The listing builds one solid part. Answer for the finished solid, in the listing's coordinates (mm). A direction names the side the tool comes from. Coordinates: 2 decimals unless noted, no trailing zeros. Order: outer loops, then holes, each group sorted by start corner. A loop starts at its lowest first (then second) coordinate and runs counter-clockwise, first axis right, second up.
from build123d import *

# Parameters (mm, degrees)
SKETCH_W        = 116
SKETCH_H        = 42
PAD_DEPTH       = 42
SKETCH005_W     = 110
SKETCH005_H     = 36
POCKET_DEPTH    = 35
SKETCH006_R     = 1.75
SKETCH006_R_2   = 15
POCKET001_DEPTH = 7.001
POCKET002_DEPTH = 5
SKETCH007_R     = 13
POCKET003_DEPTH = 42.001
SKETCH008_R     = 14
POCKET004_DEPTH = 116.001
SKETCH012_R     = 4
POCKET005_DEPTH = 5
SKETCH013_R     = 4
POCKET006_DEPTH = 5


with BuildPart() as part:
    # Sketch → Pad (new body)
    with BuildSketch(Plane.XZ):
        with Locations((0, 21)):
            Rectangle(SKETCH_W, SKETCH_H)
    extrude(amount=PAD_DEPTH)

    # Sketch005 → Pocket (cut)
    with BuildSketch(Plane(origin=(0, 0, 42), x_dir=(-1, 0, 0), z_dir=(0, 0, 1))):
        with Locations((0, 21)):
            Rectangle(SKETCH005_W, SKETCH005_H)
    extrude(amount=-POCKET_DEPTH, mode=Mode.SUBTRACT)

    # Sketch006 → Pocket001 (cut, through all)
    with BuildSketch(Plane(origin=(0, 0, 7), x_dir=(-1, 0, 0), z_dir=(0, 0, 1))):
        with Locations((-40, 33.5)):
            Circle(SKETCH006_R)
        with Locations((40, 33.5)):
            Circle(SKETCH006_R)
        with Locations((-40, 9)):
            Circle(SKETCH006_R)
        with Locations((40, 9)):
            Circle(SKETCH006_R)
        with Locations((-20, 21)):
            Circle(SKETCH006_R_2)
        with Locations((20, 21)):
            Circle(SKETCH006_R_2)
    extrude(amount=-POCKET001_DEPTH, mode=Mode.SUBTRACT)

    # Sketch011 → Pocket002 (cut)
    with BuildSketch(Plane(origin=(0, 0, 7), x_dir=(-1, 0, 0), z_dir=(0, 0, 1))):
        Polygon((-42.373287, 37.679591), (-37.615921, 37.679591), (-35.237238, 33.559591), (-37.615921, 29.439591), (-42.373287, 29.439591), (-44.75197, 33.559591), align=None)
        Polygon((37.627177, 37.64135), (42.384544, 37.64135), (44.763227, 33.52135), (42.384544, 29.40135), (37.627177, 29.40135), (35.248494, 33.52135), align=None)
        Polygon((37.575129, 13.14135), (42.332495, 13.14135), (44.711178, 9.02135), (42.332495, 4.90135), (37.575129, 4.90135), (35.196446, 9.02135), align=None)
        Polygon((-42.367844, 13.179591), (-37.610478, 13.179591), (-35.231795, 9.059591), (-37.610478, 4.939591), (-42.367844, 4.939591), (-44.746527, 9.059591), align=None)
    extrude(amount=-POCKET002_DEPTH, mode=Mode.SUBTRACT)

    # Sketch007 → Pocket003 (cut, through all)
    with BuildSketch(Plane(origin=(0, 0, 0), x_dir=(1, 0, 0), z_dir=(0, 1, 0))):
        with Locations((-24, -25)):
            Circle(SKETCH007_R)
        with Locations((7, -25)):
            Circle(SKETCH007_R)
        with Locations((38, -25)):
            Circle(SKETCH007_R)
        with BuildLine():
            ThreePointArc((-43, -16.999991), (-48, -12), (-53, -16.999992))
            Line((-53, -16.999992), (-53, -33.999979))
            ThreePointArc((-53, -33.999979), (-48, -39), (-43, -33.999978))
            Line((-43, -16.999991), (-43, -33.999978))
        make_face()
    extrude(amount=-POCKET003_DEPTH, mode=Mode.SUBTRACT)

    # Sketch008 → Pocket004 (cut, through all)
    with BuildSketch(Plane(origin=(-58, 0, 0), x_dir=(0, 0, -1), z_dir=(-1, 0, 0))):
        with Locations((-23, 22)):
            Circle(SKETCH008_R)
    extrude(amount=-POCKET004_DEPTH, mode=Mode.SUBTRACT)

    # Sketch012 → Pocket005 (cut)
    with BuildSketch(Plane(origin=(0, 0, 0), x_dir=(1, 0, 0), z_dir=(0, 1, 0))):
        with Locations((-10, 0)):
            Circle(SKETCH012_R)
        with Locations((10, 0)):
            Circle(SKETCH012_R)
    extrude(amount=-POCKET005_DEPTH, mode=Mode.SUBTRACT)

    # Sketch013 → Pocket006 (cut)
    with BuildSketch(Plane.XZ.offset(42)):
        with Locations((-10, 0)):
            Circle(SKETCH013_R)
        with Locations((10, 0)):
            Circle(SKETCH013_R)
    extrude(amount=-POCKET006_DEPTH, mode=Mode.SUBTRACT)


solid = part.part
1) Section C-C (z = 32.5) is taken. Give the number of separate pieces and of enclosed holes in the cut face, then the cut area to 3 significant figures.
2) Each of these flat-tipped pins is pushed along its axis until it touches: P1, Ø5, axis at x = 40, z = 33.5, coming from the +Y side; P2, Ø9, axis at x = 38.5, y = -8.5, coming from the +Z side; P3, Ø2, axis at x = 10.5, z = 1, coming from the +Y side. Where does it stop, or does it pass through?
3) A tool of negligible diameter and unlimited length cuts with its end or side. For faces 3 (the face through (-48, -1, 39)), 4 (the face through (43.574, -11.091, 4.535)), 5 (the face through (10, -2, 4)), from which of +Z, -Z, +X, -X, +Y, -Y can it reach the whole face along a straight path? Write none if from no direction.
4) Determine the mould class of faces 1 (the face through (-12, -1, 30)), 2 (the face through (-36.454, -31.433, 4.535)) for opening direction Y: released by +Y, released by -Y, zero draft, split by the parting line, or undercut.
5) Consider L1, parallel to X at y = -20.5, z = 2.5; L2, parallel to Y at x = 40, z = 1; L3, parallel to Y at x = 2, z = 40. Determine where each line is inside the solid, lowest interval first.
6) Section A-A (x = -48) is taken. Give the vertices of the cut face in (y, z), then the cut area to 3 significant figures.
7) Section B-B (x = -24) is taken. Give the vertices of the cut face in (y, z), then the cut area to 3 significant figures.
Filled sheet:
1. separate pieces: 10
1. enclosed holes: 0
1. area: 346 mm2
2. P1: passes through
2. P2: stops at z = 7
2. P3: stops at y = -5
3. face 3: +Y, -Y
3. face 4: +Z
3. face 5: -Z, +Y
4. face 1: zero draft
4. face 2: undercut
5. L1: x = -58 to -34.99, -5.01 to 5.01, 34.99 to 58
5. L2: y = -42 to -35.25, -31.75 to -10.75, -7.25 to 0
5. L3: y = -42 to -39, -3 to 0
6. outline: (-42, 0) - (0, 0) - (0, 12) - (-3, 12) - (-3, 7) - (-39, 7) - (-39, 12) - (-42, 12) - close; (-42, 39) - (-39, 39) - (-39, 42) - (-42, 42) - close; (-3, 39) - (0, 39) - (0, 42) - (-3, 42) - close
6. area: 342 mm2
7. outline: (-42, 0) - (-35.46, 0) - (-35.46, 7) - (-39, 7) - (-39, 12) - (-42, 12) - close; (-42, 38) - (-39, 38) - (-39, 42) - (-42, 42) - close; (-6.54, 0) - (0, 0) - (0, 12) - (-3, 12) - (-3, 7) - (-6.54, 7) - close; (-3, 38) - (0, 38) - (0, 42) - (-3, 42) - close
7. area: 146 mm2
